Geometry: final body of the model. Coordinates: model frame, mm. Face numbers are marked on the shaded views. Coordinates: 2 decimals unless noted, no trailing zeros. Loops run counter-clockwise (first coordinate to the right, second up) from the corner with the lowest first, then second, coordinate; pieces in that order, holes last. Notation, with made-up numbers: (73.5, 85.5) -> (91.5, 85.5) arc R26 ccw to (91.5, 112.5) -> close; hole circle Ø7 at (-4, 35). An arc over 180 degrees is marked (long way). One line per item, written item: value. Start each with the question number.
Item 1: Section query C-C on x = 19.5. Return loops of the section in (y, z) (3 decimals).
Item 2: Section query B-B on z = -68. Return loops of the section in (x, y) (3 decimals).
Item 3: Contact query for flat-ended pins moving along their axis: pin 1 Ø2.5 at (x, y) = (-19.5, 23.5) entering from +Z; pin 2 Ø1.6 at (x, y) = (-15.5, 20) entering from +Z; pin 3 Ø1 at (x, y) = (-15.5, 20) entering from -Z; pin 4 Ø3 at (x, z) = (7.5, -83.5) entering from +Y (3 decimals). Output: stop coordinate, or through.
Item 4: Mould query, pull axis X, two halves, no side actions, for the marked faces 1, 2 and 3. Classes: +X half, -X half, draft (parallel to the pull), parting line (faces both ways), or undercut.
Item 5: Section query D-D on z = -21. Return loops of the section in (x, y) (3 decimals).
Item 6: Section query A-A on y = 12.25. Return loops of the section in (x, z) (3 decimals).
Item 7: Ray query, probe 1 along X at (y, z) = (18.75, -129); probe 2 along Z at (x, y) = (-17, 20.5); probe 3 along Y at (x, z) = (10.5, -60.5) (3 decimals). Return the intervals inside material, ascending. Write a range as from..to.
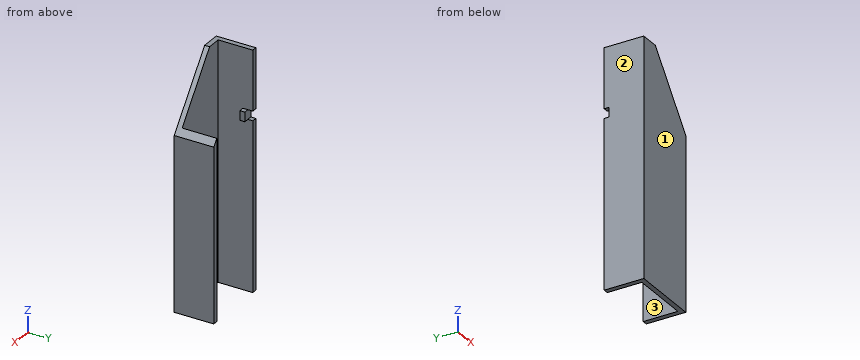
Autodesk Inventor part; units mm, degrees
ref_plane "YZ Plane" through (0, 0, 0) normal (1, 0, 0) x (0, 1, 0)
ref_plane "XZ Plane" through (0, 0, 0) normal (0, 1, 0) x (-1, 0, 0)
ref_plane "XY Plane" through (0, 0, 0) normal (0, 0, 1) x (1, 0, 0)
sketch "Sketch1" plane through (0, 0, 0) normal (0, 0, 1) x (1, 0, 0)
  line L0 (24.1101, 25.4) -> (24.1101, 0)
  line L1 (24.1101, 0) -> (-20.3399, 0)
  line L2 (-20.3399, 0) -> (-20.3399, 25.4)
  line L3 (-17.1649, 25.4) -> (-17.1649, 3.175)
  line L4 (-17.1649, 3.175) -> (20.9351, 3.175)
  line L5 (20.9351, 3.175) -> (20.9351, 25.4)
  line L6 (-20.3399, 25.4) -> (-17.1649, 25.4)
  line L7 (24.1101, 25.4) -> (20.9351, 25.4)
  point P0 (0, 0)
  dimension "d0" = 44.45
  dimension "d1" = 25.4
  dimension "d2" = 3.175
extrude "Extrusion1" add sketch "Sketch1" against normal blind 152.4
sketch "Sketch3" plane through (-20.3399, 0, 0) normal (-1, 0, 0) x (0, 0, 1)
  line L0 (0, 25.4) -> (-152.4, 25.4)
  line L1 (-152.4, 0) -> (-152.4, 25.4)
  line L2 (0, 0) -> (-152.4, 0)
  line L3 (-44.45, 25.4) -> (-44.45, 19.05)
  line L4 (-44.45, 19.05) -> (-38.354, 19.05)
  line L5 (-38.354, 19.05) -> (-38.354, 25.4)
  dimension "d6" = 6.096
  dimension "d7" = 6.35
  dimension "d8" = 107.95
extrude "Extrusion2" cut sketch "Sketch3" against normal up to next
sketch "Sketch4" plane through (-20.3399, 0, 0) normal (-1, 0, 0) x (0, 0, 1)
  line L0 (-38.354, 19.05) -> (-44.45, 19.05)
  line L1 (-44.45, 19.05) -> (-44.45, 22.225)
  line L2 (-44.45, 25.4) -> (-44.45, 19.05)
  line L3 (-38.354, 19.05) -> (-38.354, 25.4)
  line L4 (-38.354, 19.05) -> (-44.45, 19.05)
  line L5 (-44.45, 19.05) -> (-38.354, 19.05)
  line L6 (-44.45, 22.225) -> (-38.354, 22.225)
  line L7 (-38.354, 19.05) -> (-38.354, 22.225)
  dimension "d11" = 3.175
extrude "Extrusion3" add sketch "Sketch4" against normal blind 6.35
sketch "Sketch5" plane through (-20.3399, 0, 0) normal (0, -1, 0) x (1, 0, 0)
  line L0 (0, 0) -> (44.45, 0)
  line L1 (44.45, 0) -> (44.45, -152.4)
  line L2 (44.45, -152.4) -> (44.45, -41.275)
  line L3 (44.45, 0) -> (44.45, -152.4)
  line L4 (44.45, -41.275) -> (12.2024, 0)
  line L5 (12.2024, 0) -> (44.45, 0)
  line L6 (44.45, 0) -> (44.45, -41.275)
  point P0 (20.3399, 0)
  dimension "d14" = 111.125
  dimension "d15" = 38
extrude "Extrusion4" cut sketch "Sketch5" against normal through all
properties part number "Horizontal channel"
Reply:
1. outline: (0, -152.4) -> (3.175, -152.4) -> (3.175, -35.374) -> (0, -35.374) -> close
2. outline: (-20.34, 0) -> (24.11, 0) -> (24.11, 25.4) -> (20.935, 25.4) -> (20.935, 3.175) -> (-17.165, 3.175) -> (-17.165, 25.4) -> (-20.34, 25.4) -> close
3. pin 1: stops at z = 0
3. pin 2: stops at z = -38.35
3. pin 3: stops at z = -44.45
3. pin 4: stops at y = 3.175
4. face 1: draft
4. face 2: -X half
4. face 3: undercut
5. outline: (-20.34, 0) -> (8.27, 0) -> (8.27, 3.175) -> (-17.165, 3.175) -> (-17.165, 25.4) -> (-20.34, 25.4) -> close
6. outline: (-20.34, -152.4) -> (-17.165, -152.4) -> (-17.165, 0) -> (-20.34, 0) -> close; (20.935, -152.4) -> (24.11, -152.4) -> (24.11, -41.275) -> (20.935, -37.211) -> close
7. probe 1: x = -20.34..-17.16, 20.94..24.11
7. probe 2: z = -44.45..-38.35
7. probe 3: y = 0..3.175
